The listing builds one solid part. Answer for the finished solid, in the listing's coordinates (mm). Round coordinates to 2 decimals unless told otherwise and drop trailing zeros. Write each question's results on one line, items separated by ' | '. Start each with the question number.
(1) A flat-ended cylindrical pin translates along its axis: pin 1 (2 mm diameter, centred on x = -45.24, y = -23.5, fed in from -Z). Find the tip coordinate at first contact, or state that the pin passes through.
(2) Straight lines are drawn through the part: probe 1 along Y at (x, z) = (131, 2.5); probe 2 along Y at (x, z) = (133, 1.65); probe 3 along Z at (x, y) = (3.5, 0). For each, find the intervals that lie inside material, in ascending order.
(3) Determine the mould class of faces 1 (the face through (-137.52, 10.83, 2.72)), 2 (the face through (-2, -38, 0)) for opening direction Y: released by +Y, released by -Y, zero draft, split by the parting line, or undercut.
```python
from build123d import *

# Parameters (mm, degrees)
BOSS_EXTRU_1_DEPTH           = 5
ESQUISSE2_R                  = 2.5
ENL_V_MAT_EXTRU_1_DEPTH      = 5
ESQUISSE3_R                  = 0.5
ENL_V_MAT_EXTRU_2_DEPTH      = 1
ENL_V_MAT_EXTRU_2_DEPTH_BACK = 311
ESQUISSE4_R                  = 1.75
ENL_V_MAT_EXTRU_3_DEPTH      = 5
ESQUISSE6_R                  = 3
ENL_V_MAT_EXTRU_4_DEPTH      = 5
CONG_1_R                     = 0.5


with BuildPart() as part:
    # Esquisse1 → Boss.-Extru.1 (new body)
    with BuildSketch(Plane.XY):
        with BuildLine():
            Line((-153.5, -68.5), (153.5, -68.5))
            ThreePointArc((153.5, -68.5), (154.560660172, -68.060660172), (155, -67))
            Line((155, -67), (155, 67))
            ThreePointArc((155, 67), (154.560660172, 68.060660172), (153.5, 68.5))
            Line((153.5, 68.5), (-153.5, 68.5))
            ThreePointArc((-153.5, 68.5), (-154.560660172, 68.060660172), (-155, 67))
            Line((-155, 67), (-155, -67))
            ThreePointArc((-155, -67), (-154.560660172, -68.060660172), (-153.5, -68.5))
        make_face()
    extrude(amount=BOSS_EXTRU_1_DEPTH)

    # Esquisse2 → Enlèv. mat.-Extru.1 (cut)
    with BuildSketch(Plane(origin=(0, 0, 0), x_dir=(-1, 0, 0), z_dir=(0, 0, -1))):
        with Locations((-131.119201541, -60)):
            Circle(ESQUISSE2_R)
        with Locations((-131.119201541, 60)):
            Circle(ESQUISSE2_R)
        with Locations((131.119201541, 60)):
            Circle(ESQUISSE2_R)
        with Locations((131.119201541, -60)):
            Circle(ESQUISSE2_R)
    extrude(amount=-ENL_V_MAT_EXTRU_1_DEPTH, mode=Mode.SUBTRACT)

    # Esquisse3 → Enlèv. mat.-Extru.2 (cut, two sides)
    with BuildSketch(Plane(origin=(155, 0, 0), x_dir=(0, 0, -1), z_dir=(1, 0, 0))) as enl_v_mat_extru_2_sk:
        Circle(ESQUISSE3_R)
        with Locations((0, 2)):
            Circle(ESQUISSE3_R)
        with Locations((0, 4)):
            Circle(ESQUISSE3_R)
        with Locations((0, 6)):
            Circle(ESQUISSE3_R)
        with Locations((0, 8)):
            Circle(ESQUISSE3_R)
        with Locations((0, -2)):
            Circle(ESQUISSE3_R)
        with Locations((0, -4)):
            Circle(ESQUISSE3_R)
        with Locations((0, -6)):
            Circle(ESQUISSE3_R)
        with Locations((0, -8)):
            Circle(ESQUISSE3_R)
    extrude(amount=ENL_V_MAT_EXTRU_2_DEPTH, mode=Mode.SUBTRACT)
    extrude(enl_v_mat_extru_2_sk.sketch, amount=-ENL_V_MAT_EXTRU_2_DEPTH_BACK, mode=Mode.SUBTRACT)

    # Esquisse4 → Enlèv. mat.-Extru.3 (cut)
    with BuildSketch(Plane(origin=(0, 0, 0), x_dir=(-1, 0, 0), z_dir=(0, 0, -1))):
        with Locations((45.235873588, -23.5)):
            Circle(ESQUISSE4_R)
        with Locations((123.985873588, 23.5)):
            Circle(ESQUISSE4_R)
    extrude(amount=-ENL_V_MAT_EXTRU_3_DEPTH, mode=Mode.SUBTRACT)

    # Esquisse6 → Enlèv. mat.-Extru.4 (cut)
    with BuildSketch(Plane(origin=(0, 0, 0), x_dir=(-1, 0, 0), z_dir=(0, 0, -1))):
        with Locations((134.746454325, 11.977670931)):
            Circle(ESQUISSE6_R)
    extrude(amount=-ENL_V_MAT_EXTRU_4_DEPTH, mode=Mode.SUBTRACT)

    # Congé1
    cong_1_edges = [part.edges().sort_by_distance(p)[0] for p in [
        (-131.746454325, 11.977670931, 0),
    ]]
    fillet(cong_1_edges, radius=CONG_1_R)


solid = part.part
```
Checked values:
1) pin 1: passes through
2) probe 1: y = -68.5 to -62.5, -57.5 to 57.5, 62.5 to 68.5 | probe 2: y = -68.5 to -61.65, -58.35 to 58.35, 61.65 to 68.5 | probe 3: z = 0.5 to 5
3) face 1: undercut | face 2: zero draft
